The listing builds one solid part. Answer for the finished solid, in the listing's coordinates (mm). A direction names the side the tool comes from. Give positions to 0.01 mm unless a question says otherwise; leave off trailing zeros. Order: outer loops, then holes, each group sorted by start corner. A loop starts at its lowest first (then second) coordinate and runs counter-clockwise, first axis right, second up. Notation, with made-up numbers: (63, -36.75) - (77, -36.75) arc R18 cw to (77, -19.75) - close; hole circle Ø3 at (40.5, 13). An arc over 180 degrees is marked (long way). Use a Markdown table: item, result. Add a question column.
1) Find section C-C, the plane y = 129. Determine the outline of the cut face in (x, z).
2) Flat-ended cylindrical pins translate along their axes: pin 1 (4 mm diameter, centred on x = -258, z = 4.5, fed in from -Y); pin 2 (3.5 mm diameter, centred on y = 162.5, z = 2, fed in from +X); pin 3 (4.5 mm diameter, centred on y = 172, z = 5.5, fed in from +X); pin 4 (5 mm diameter, centred on x = -231.5, y = 162.5, fed in from -Z). Find the tip coordinate at first contact, or state that the pin passes through.
3) The mould has two halves that part along Y. Classify faces 6 (the face through (-205, 147.65, 4)), 7 (the face through (-138.424, 154, 4)), 8 (the face through (-295.34, 173.12, 4.26)), 9 (the face through (-287.156, 166.404, 4.17)): released by +Y, released by -Y, zero draft, split by the parting line, or undercut.
4) For faces 1 (the face through (-278, 179.4, 4)), 2 (the face through (-235, 148, 0)), 3 (the face through (-276.847, 106, 3)), 4 (the face through (-203, 160.35, 4)), 5 (the face through (-268.897, 113, 3)), determine the directions among +Z, -Z, +X, -X, +Y, -Y from which every point of the face is accessible in a straight line to the end or side of a thin tool.
5) Find section A-A, the plane z = 3.75. State how many separate pieces and enclosed holes the cut face has, plus the area to 3 significant figures.
6) Find section B-B, the plane x = -152. Determine the outline of the cut face in (y, z), plus the area to 3 significant figures.
7) Straight lines are drawn through the part: line 1 (X direction, y = 170, z = 7.5); line 2 (Y direction, x = -261, z = 1.75); line 3 (Z direction, x = -233.5, y = 160). For each, find the intervals that lie inside material, in ascending order.
from build123d import *

# Parameters (mm, degrees)
BOSS_EXTRUDE1_OUTLINE_R = 3.556
BOSS_EXTRUDE1_OUTLINE_W = 260.9469
BOSS_EXTRUDE1_OUTLINE_H = 138.1252
BOSS_EXTRUDE1_DEPTH     = 76.2
CUT_EXTRUDE1_DEPTH      = 355.32482824
CUT_EXTRUDE1_DEPTH_BACK = 355.32482824
FILLET1_R               = 2.54
SKETCH7_W               = 260.9469
SKETCH7_H               = 22.1996
CUT_EXTRUDE2_DEPTH      = 347.152897849
FILLET2_R               = 6.35
SKETCH8_W               = 217.439036591
SKETCH8_H               = 235.521960295
CUT_EXTRUDE4_DEPTH      = 347.144751077
SKETCH9_W               = 181.772335281
SKETCH9_H               = 128.639747743
CUT_EXTRUDE5_DEPTH      = 347.144751077


# Read off the part's stored shape, not the designer's step: Boss-Extrude1
with BuildPart() as part:
    # Boss-Extrude1 outline → Boss-Extrude1 (new body)
    with BuildSketch(Plane.XY):
        with BuildLine():
            Line((-286.3596, -22.225), (9.525, -22.225))
            ThreePointArc((9.525, -22.225), (19.05, -12.7), (9.525, -3.175))
            ThreePointArc((9.525, -3.175), (19.05, 6.35), (9.525, 15.875))
            ThreePointArc((9.525, 15.875), (2.789807909, 18.664807909), (0, 25.4))
            Line((0, 25.4), (0, 131.7752))
            ThreePointArc((0, 131.7752), (2.789807909, 138.510392091), (9.525, 141.3002))
            ThreePointArc((9.525, 141.3002), (19.05, 150.8252), (9.525, 160.3502))
            ThreePointArc((9.525, 160.3502), (19.05, 169.8752), (9.525, 179.4002))
            Line((9.525, 179.4002), (-6.35, 179.4002))
            Line((-6.35, 179.4002), (-6.35, 163.5252))
            Line((-6.35, 163.5252), (-7.9502, 163.5252))
            Line((-7.9502, 163.5252), (-7.9502, 160.3502))
            Line((-7.9502, 160.3502), (-268.9098, 160.3502))
            Line((-268.9098, 160.3502), (-268.9098, 163.5252))
            Line((-268.9098, 163.5252), (-270.51, 163.5252))
            Line((-270.51, 163.5252), (-270.51, 179.4002))
            Line((-270.51, 179.4002), (-286.385, 179.4002))
            ThreePointArc((-286.385, 179.4002), (-295.91, 169.8752), (-286.385, 160.3502))
            ThreePointArc((-286.385, 160.3502), (-295.897297883, 150.818850004), (-286.3723, 141.3002))
            ThreePointArc((-286.3723, 141.3002), (-279.637107909, 138.510392091), (-276.8473, 131.7752))
            Line((-276.8473, 131.7752), (-276.8473, 25.4))
            ThreePointArc((-276.8473, 25.4), (-279.637107909, 18.664807909), (-286.3723, 15.875))
            ThreePointArc((-286.3723, 15.875), (-295.8973, 6.35), (-286.3723, -3.175))
            ThreePointArc((-286.3723, -3.175), (-295.884597883, -12.706349996), (-286.3596, -22.225))
        make_face()
        with Locations((-286.3596, -12.7)):
            Circle(BOSS_EXTRUDE1_OUTLINE_R, mode=Mode.SUBTRACT)
        with Locations((-286.3723, 6.35)):
            Circle(BOSS_EXTRUDE1_OUTLINE_R, mode=Mode.SUBTRACT)
        with Locations((9.525, -12.7)):
            Circle(BOSS_EXTRUDE1_OUTLINE_R, mode=Mode.SUBTRACT)
        with Locations((9.525, 6.35)):
            Circle(BOSS_EXTRUDE1_OUTLINE_R, mode=Mode.SUBTRACT)
        with Locations((-286.3723, 150.8252)):
            Circle(BOSS_EXTRUDE1_OUTLINE_R, mode=Mode.SUBTRACT)
        with Locations((-286.385, 169.8752)):
            Circle(BOSS_EXTRUDE1_OUTLINE_R, mode=Mode.SUBTRACT)
        with Locations((-138.42365, 78.5876)):
            Rectangle(BOSS_EXTRUDE1_OUTLINE_W, BOSS_EXTRUDE1_OUTLINE_H, mode=Mode.SUBTRACT)
        with Locations((9.525, 150.8252)):
            Circle(BOSS_EXTRUDE1_OUTLINE_R, mode=Mode.SUBTRACT)
        with Locations((9.525, 169.8752)):
            Circle(BOSS_EXTRUDE1_OUTLINE_R, mode=Mode.SUBTRACT)
    extrude(amount=BOSS_EXTRUDE1_DEPTH)

    # Sketch5 → Cut-Extrude1 (cut, two sides: drawn at the far end of the back side and taken through both)
    with BuildSketch(Plane.ZY.offset(276.8473).offset(-CUT_EXTRUDE1_DEPTH_BACK)):
        Polygon((1.6002, -22.225), (8.641107133, 179.4002), (76.2, 179.4002), (76.2, -22.225), align=None)
    extrude(amount=CUT_EXTRUDE1_DEPTH + CUT_EXTRUDE1_DEPTH_BACK, mode=Mode.SUBTRACT)

    # Fillet1
    fillet1_edges = [part.edges().sort_by_distance(p)[0] for p in [
        (-286.385, 160.3502, 3.987933237),
        (-286.3723, -3.175, 1.132720329),
        (9.525, -3.175, 1.132720329),
        (9.525, 160.3502, 3.987933237),
    ]]
    fillet(fillet1_edges, radius=FILLET1_R)

    # Sketch7 → Cut-Extrude2 (cut, through all)
    with BuildSketch(Plane(origin=(0, 0, 0), x_dir=(-1, 0, 0), z_dir=(0, 0, -1))):
        with Locations((138.42365, -6.35)):
            Rectangle(SKETCH7_W, SKETCH7_H)
    extrude(amount=-CUT_EXTRUDE2_DEPTH, mode=Mode.SUBTRACT)

    # Fillet2
    fillet2_edges = [part.edges().sort_by_distance(p)[0] for p in [
        (-268.8971, 4.7498, 1.271090386),
        (-268.8971, -17.4498, 0.883476829),
        (-7.9502, -17.4498, 0.883476829),
        (-7.9502, 4.7498, 1.271090386),
    ]]
    fillet(fillet2_edges, radius=FILLET2_R)

    # Sketch8 → Cut-Extrude4 (cut, through all)
    with BuildSketch(Plane(origin=(0, -0.082881646, 2.373419811), x_dir=(1, 0, 0), z_dir=(0, -0.03489949670250444, 0.9993908270190958))):
        with Locations((-29.704131704, 74.917246318)):
            Rectangle(SKETCH8_W, SKETCH8_H)
    extrude(amount=-CUT_EXTRUDE4_DEPTH, mode=Mode.SUBTRACT)

    # Sketch9 → Cut-Extrude5 (cut, through all)
    with BuildSketch(Plane(origin=(0, -0.082881646, 2.373419811), x_dir=(1, 0, 0), z_dir=(0, -0.03489949670250444, 0.9993908270190958))):
        with Locations((-229.309817641, 14.398560918)):
            Rectangle(SKETCH9_W, SKETCH9_H)
    extrude(amount=-CUT_EXTRUDE5_DEPTH, mode=Mode.SUBTRACT)


solid = part.part
The answers:
| question | item | result |
|---|---|---|
| 1 | outline | (-276.85, 0) - (-268.9, 0) - (-268.9, 6.88) - (-276.85, 6.88) - close |
| 2 | pin 1 | y = 147.65 |
| 2 | pin 2 | x = -268.91 |
| 2 | pin 3 | x = -270.51 |
| 2 | pin 4 | z = 0 |
| 3 | face 6 | released by -Y |
| 3 | face 7 | zero draft |
| 3 | face 8 | undercut |
| 3 | face 9 | undercut |
| 4 | face 1 | +Z, -Z, +X, -X, +Y |
| 4 | face 2 | -Z, +X, -X, +Y, -Y |
| 4 | face 3 | +Z, -Z, -X, -Y |
| 4 | face 4 | +Z, -Z, +X, +Y |
| 4 | face 5 | +Z, -Z, +X, -Y |
| 5 | separate pieces | 1 |
| 5 | enclosed holes | 2 |
| 5 | area | 3,030 mm2 |
| 6 | outline | (147.65, 0) - (160.35, 0) - (160.35, 7.98) - (147.65, 7.53) - close |
| 6 | area | 98.5 mm2 |
| 7 | line 1 | -295.91 to -289.94, -282.83 to -270.51 |
| 7 | line 2 | 147.65 to 160.35 |
| 7 | line 3 | 0 to 7.96 |
